Read the model definition and answer for the solid it produces. Units are mm, in the model's axes. Face numbers are marked on the shaded views. A direction names the side the tool comes from. Give positions to 0.01 mm unless a question says otherwise; leave off trailing zeros. Write each loop counter-clockwise with the first axis right and the second up, starting at its lowest first coordinate (ties: lowest second). Pieces come first, ordered by that corner, then holes. Notation, with made-up numbers: (-35.75, 53.25) -> (2.25, 53.25) arc R7 cw to (2.25, 57.25) -> close; hole circle Ø11 at (-29, 9.5). An arc over 180 degrees is marked (long way). Write item = value, one per line.
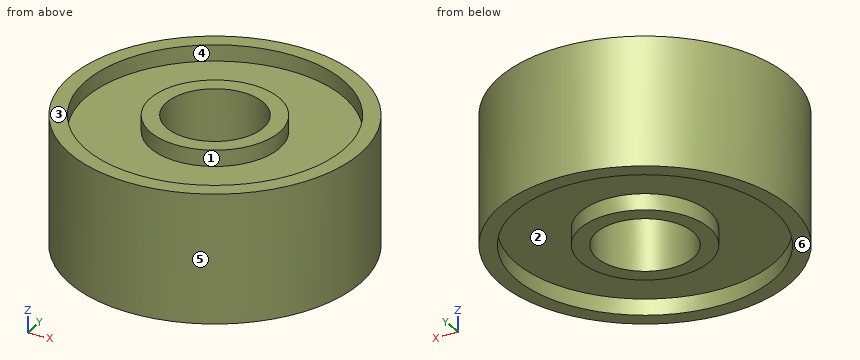
from build123d import *

# Parameters (mm, degrees)
SKETCH_1_R          = 4.5
EXTRUDE_1_DEPTH     = 2
SKETCH_2_R          = 1.5
CUT_EXTRUDE_1_DEPTH = 5
SKETCH_3_R          = 4
SKETCH_3_R_2        = 2
CUT_EXTRUDE_2_DEPTH = 0.5


with BuildPart() as part:
    # 草圖1 → 填料-伸長1 (new body, symmetric)
    with BuildSketch(Plane.XY):
        Circle(SKETCH_1_R)
    extrude(amount=EXTRUDE_1_DEPTH, both=True)

    # 草圖2 → 除料-伸長1 (cut, through all)
    with BuildSketch(Plane.XY.offset(2)):
        Circle(SKETCH_2_R)
    extrude(amount=-CUT_EXTRUDE_1_DEPTH, mode=Mode.SUBTRACT)

    # 草圖3 → 除料-伸長2 (cut)
    with BuildSketch(Plane.XY.offset(2)):
        Circle(SKETCH_3_R)
        Circle(SKETCH_3_R_2, mode=Mode.SUBTRACT)
    cut_extrude_2 = extrude(amount=-CUT_EXTRUDE_2_DEPTH, mode=Mode.SUBTRACT)

    # 鏡射1: 除料-伸長2 across plane
    add(cut_extrude_2.mirror(Plane.XY), mode=Mode.SUBTRACT)


solid = part.part
(1) For a pull along X with two mould halves and no side action, classify the marked faces 4, 5 and 6 as released by +X, released by -X, zero draft, split by the parting line, or undercut.
Checks:
face_4 = undercut
face_5 = split by the parting line
face_6 = zero draft
(2) The part is cut by section C-C on z = -0.55. Determine the outline of the cut face in (x, y), plus the area to 3 significant figures.
Checks:
outline = circle Ø9 at (0, 0); hole circle Ø3 at (0, 0)
area = 56.5 mm²
(3) The part is cut by section A-A on x = 0. Determine the outline of the cut face in (y, z).
Checks:
outline = (-4.5, -2) -> (-4, -2) -> (-4, -1.5) -> (-2, -1.5) -> (-2, -2) -> (-1.5, -2) -> (-1.5, 2) -> (-2, 2) -> (-2, 1.5) -> (-4, 1.5) -> (-4, 2) -> (-4.5, 2) -> close; (1.5, -2) -> (2, -2) -> (2, -1.5) -> (4, -1.5) -> (4, -2) -> (4.5, -2) -> (4.5, 2) -> (4, 2) -> (4, 1.5) -> (2, 1.5) -> (2, 2) -> (1.5, 2) -> close
(4) Consider L1, parallel to Z at x = -2, y = 0.5; L2, parallel to Y at x = 1, z = -0.8; L3, parallel to X at y = -1.25, z = -0.1. Determine where each line is inside the solid, lowest interval first.
Checks:
L1 = -1.5 to 1.5
L2 = -4.39 to -1.12, 1.12 to 4.39
L3 = -4.32 to -0.83, 0.83 to 4.32
(5) The part is cut by section D-D on y = 3.25. Determine the outline of the cut face in (x, z), plus the area to 3 significant figures.
Checks:
outline = (-3.11, -2) -> (-2.33, -2) -> (-2.33, -1.5) -> (2.33, -1.5) -> (2.33, -2) -> (3.11, -2) -> (3.11, 2) -> (2.33, 2) -> (2.33, 1.5) -> (-2.33, 1.5) -> (-2.33, 2) -> (-3.11, 2) -> close
area = 20.2 mm²
(6) Given P1, Ø2.5, axis at x = 2, y = -1, coming from the -Z side; P2, Ø1.5, axis at x = 3, z = -0.5, coming from the -Y side, each flat-ended and moving along its own axis, determine where each tip first touches the part or whether it passes through.
Checks:
P1 = -2
P2 = -3.9
(7) A tool of negligible diameter and unlimited length cuts with its end or side. For the marked faces 1, 2 and 3, from which of +Z, -Z, +X, -X, +Y, -Y can it reach the whole face along a straight path? Write none if from no direction.
Checks:
face_1 = +Z
face_2 = -Z
face_3 = +Z, +X, -X, +Y, -Y
